Model file for the job. Use its own axes, mm. A direction names the side the tool comes from. Coordinates: 2 decimals unless noted, no trailing zeros. Write each loop counter-clockwise with the first axis right and the second up, starting at its lowest first coordinate (ties: lowest second). Pieces come first, ordered by that corner, then holes. Notation, with made-up numbers: (53, 65) - (103, 65) arc R30 cw to (103, 92) - close; hole circle Ø11 at (49.25, 62.5). An arc over 180 degrees is marked (long way). Put each result on its own line as item: value. Start each with the question number.
1. Pull direction X, two halves, no side cores. Call faces 3 (the face through (0.5, 5.32, 2.23)), 4 (the face through (2, 4.318, -2)), 5 (the face through (-26.67, 3, 0)), 6 (the face through (25.584, 3.131, 15.364)): released by +X, released by -X, zero draft, split by the parting line, or undercut.
2. Saw through at D-D, the plane y = 0.75. Write the cut outline in (x, z).
3. Which spindle directions (+Z, -Z, +X, -X, +Y, -Y) get a long thin tool onto all of the face, cutting with end or side? Do faces 1 (the face through (-0.83, 2.13, -3.72)), 2 (the face through (22.1, 3.1, 13.2)). Say none if no direction does.
4. Saw through at B-B, the plane z = 0. Write the cut outline in (x, y), plus the area to 3 significant figures.
5. Saw through at C-C, the plane y = 5.75. Write the cut outline in (x, z).
6. Drill centre lines: L1, parallel to Z at x = 0, y = 5.1; L2, parallel to X at y = 5.1, z = 0; L3, parallel to X at y = 5.5, z = -12.5. Where is each one in solid material? Low to high. Write a range as from..to.
7. Saw through at A-A, the plane x = 0. Write the cut outline in (y, z).
8. Drop flat-ended pins along their axis: P1, Ø3, axis at x = 23.241, z = 13.208, coming from the +Y side; P2, Ø7, axis at x = 0, z = 0, coming from the -Y side. Give the stop position or say it passes through.
```python
from build123d import *

# Parameters (mm, degrees)
SKETCH1_R           = 1.143
BOSS_EXTRUDE1_DEPTH = 6.35
SKETCH2_R           = 3.81
CUT_EXTRUDE1_DEPTH  = 4.318
SKETCH3_R           = 2.286
CUT_EXTRUDE2_DEPTH  = 4.318


with BuildPart() as part:
    # Sketch1 → Boss-Extrude1 (new body)
    with BuildSketch(Plane(origin=(0, 0, 0), x_dir=(1, 0, 0), z_dir=(0, 1, 0))):
        with BuildLine():
            Line((-22.86, 16.51), (22.86, 16.51))
            ThreePointArc((22.86, 16.51), (25.554076836, 15.394076836), (26.67, 12.7))
            Line((26.67, 12.7), (26.67, -12.7))
            ThreePointArc((26.67, -12.7), (25.554076836, -15.394076836), (22.86, -16.51))
            Line((22.86, -16.51), (18.7325, -16.51))
            Line((18.7325, -16.51), (-18.7325, -16.51))
            Line((-18.7325, -16.51), (-22.86, -16.51))
            ThreePointArc((-22.86, -16.51), (-25.554076836, -15.394076836), (-26.67, -12.7))
            Line((-26.67, -12.7), (-26.67, 12.7))
            ThreePointArc((-26.67, 12.7), (-25.554076836, 15.394076836), (-22.86, 16.51))
        make_face()
        with Locations((-23.241, 13.208)):
            Circle(SKETCH1_R, mode=Mode.SUBTRACT)
        with Locations((23.241, 13.208)):
            Circle(SKETCH1_R, mode=Mode.SUBTRACT)
        with Locations((23.241, -13.208)):
            Circle(SKETCH1_R, mode=Mode.SUBTRACT)
        with Locations((-23.50753981, -13.208)):
            Circle(SKETCH1_R, mode=Mode.SUBTRACT)
    extrude(amount=BOSS_EXTRUDE1_DEPTH)

    # Sketch2 → Cut-Extrude1 (cut)
    with BuildSketch(Plane.XZ):
        Circle(SKETCH2_R)
    extrude(amount=-CUT_EXTRUDE1_DEPTH, mode=Mode.SUBTRACT)

    # Sketch3 → Cut-Extrude2 (cut)
    with BuildSketch(Plane(origin=(0, 4.318, 0), x_dir=(-1, 0, 0), z_dir=(0, -1, 0))):
        Circle(SKETCH3_R)
    extrude(amount=-CUT_EXTRUDE2_DEPTH, mode=Mode.SUBTRACT)


solid = part.part
```
Final values:
1. face 3: undercut
1. face 4: undercut
1. face 5: released by -X
1. face 6: released by +X
2. outline: (-26.67, -12.7) arc R3.81 ccw to (-22.86, -16.51) - (22.86, -16.51) arc R3.81 ccw to (26.67, -12.7) - (26.67, 12.7) arc R3.81 ccw to (22.86, 16.51) - (-22.86, 16.51) arc R3.81 ccw to (-26.67, 12.7) - close; hole circle Ø2.29 at (-23.51, 13.21); hole circle Ø2.29 at (-23.24, -13.21); hole circle Ø7.62 at (0, 0); hole circle Ø2.29 at (23.24, -13.21); hole circle Ø2.29 at (23.24, 13.21)
3. face 1: -Y
3. face 2: +Y, -Y
4. outline: (-26.67, 0) - (-3.81, 0) - (-3.81, 4.32) - (-2.29, 4.32) - (-2.29, 6.35) - (-26.67, 6.35) - close; (2.29, 4.32) - (3.81, 4.32) - (3.81, 0) - (26.67, 0) - (26.67, 6.35) - (2.29, 6.35) - close
4. area: 297 mm²
5. outline: (-26.67, -12.7) arc R3.81 ccw to (-22.86, -16.51) - (22.86, -16.51) arc R3.81 ccw to (26.67, -12.7) - (26.67, 12.7) arc R3.81 ccw to (22.86, 16.51) - (-22.86, 16.51) arc R3.81 ccw to (-26.67, 12.7) - close; hole circle Ø2.29 at (-23.51, 13.21); hole circle Ø2.29 at (-23.24, -13.21); hole circle Ø4.57 at (0, 0); hole circle Ø2.29 at (23.24, -13.21); hole circle Ø2.29 at (23.24, 13.21)
6. L1: z = -16.51..-2.29, 2.29..16.51
6. L2: x = -26.67..-2.29, 2.29..26.67
6. L3: x = -26.67..-24.14, -22.34..22.34, 24.14..26.67
7. outline: (0, -16.51) - (6.35, -16.51) - (6.35, -2.29) - (4.32, -2.29) - (4.32, -3.81) - (0, -3.81) - close; (0, 3.81) - (4.32, 3.81) - (4.32, 2.29) - (6.35, 2.29) - (6.35, 16.51) - (0, 16.51) - close
8. P1: stops at y = 6.35
8. P2: stops at y = 4.32
